from build123d import *

# Parameters (mm, degrees)
CROQUIS1_W                   = 15
CROQUIS1_H                   = 9
CROQUIS1_W_2                 = 13
CROQUIS1_H_2                 = 7
SALIENTE_EXTRUIR1_DEPTH      = 9
CROQUIS2_W                   = 15
CROQUIS2_H                   = 9
SALIENTE_EXTRUIR2_DEPTH      = 0.1
CROQUIS3_W                   = 3
CROQUIS3_H                   = 3.407555274
CORTAR_EXTRUIR1_DEPTH        = 7
CROQUIS4_W                   = 0.7
CROQUIS4_H                   = 0.7
SALIENTE_EXTRUIR3_DEPTH      = 3.5
SALIENTE_EXTRUIR3_DEPTH_BACK = 6


with BuildPart() as part:
    # Croquis1 → Saliente-Extruir1 (new body)
    with BuildSketch(Plane.XY):
        Rectangle(CROQUIS1_W, CROQUIS1_H)
        Rectangle(CROQUIS1_W_2, CROQUIS1_H_2, mode=Mode.SUBTRACT)
    extrude(amount=SALIENTE_EXTRUIR1_DEPTH)

    # Croquis2 → Saliente-Extruir2 (add)
    with BuildSketch(Plane(origin=(0, 0, 0), x_dir=(-1, 0, 0), z_dir=(0, 0, -1))):
        Rectangle(CROQUIS2_W, CROQUIS2_H)
    extrude(amount=SALIENTE_EXTRUIR2_DEPTH)

    # Croquis3 → Cortar-Extruir1 (cut)
    with BuildSketch(Plane.XY.offset(9)):
        with Locations((0, 3.5)):
            Rectangle(CROQUIS3_W, CROQUIS3_H)
    extrude(amount=-CORTAR_EXTRUIR1_DEPTH, mode=Mode.SUBTRACT)

    # Croquis4 → Saliente-Extruir3 (add, two sides)
    with BuildSketch(Plane(origin=(0, 0, -0.1), x_dir=(-1, 0, 0), z_dir=(0, 0, -1))) as saliente_extruir3_sk:
        with Locations((-2.15, 1.15)):
            Rectangle(CROQUIS4_W, CROQUIS4_H)
        with Locations((0.39, 1.15)):
            Rectangle(CROQUIS4_W, CROQUIS4_H)
        with Locations((2.93, 1.15)):
            Rectangle(CROQUIS4_W, CROQUIS4_H)
        with Locations((0.39, -1.39)):
            Rectangle(CROQUIS4_W, CROQUIS4_H)
        with Locations((2.93, -1.39)):
            Rectangle(CROQUIS4_W, CROQUIS4_H)
        with Locations((-2.15, -1.39)):
            Rectangle(CROQUIS4_W, CROQUIS4_H)
    extrude(amount=SALIENTE_EXTRUIR3_DEPTH)
    extrude(saliente_extruir3_sk.sketch, amount=-SALIENTE_EXTRUIR3_DEPTH_BACK)


solid = part.part
Here's how the part is built. I have some questions about the finished solid (model axes, mm). A direction names the side the tool comes from. Coordinates: 2 decimals unless noted, no trailing zeros. Loops run counter-clockwise (first coordinate to the right, second up) from the corner with the lowest first, then second, coordinate; pieces in that order, holes last.
1. For P1, Ø1, axis at x = 5, y = 2.5, coming from the -Z side; P2, Ø0.8, axis at y = 1, z = -2.5, coming from the -X side; P3, Ø0.8, axis at x = -0.5, z = 2.5, coming from the +Y side, each with a flat end and sliding along its axis, tell me the tip position at first contact or that it passes through.
2. For faces 1 (the flat face through (0, -4, 9)), 2 (the flat face through (0, 4, 2)), 3 (the flat face through (0, -3.5, 4)), which set-ups out of +Z, -Z, +X, -X, +Y, -Y let a thin tool reach every point of the face, with its end or its side?
3. Imagine slicing it at D-D, the plane z = -1.25. Please give me the cut outline in (x, y).
4. Imagine slicing it at B-B, the plane x = 6. Please give me the cut outline in (y, z), and give its area (3 significant figures).
5. If we mould it in two halves opening along Y, with no side actions, what happens to faces 4 (the flat face through (-6.5, 0, 4)), 5 (the flat face through (1.5, 4, 6)), 6 (the flat face through (0, -4.5, 5))? For each: pulls with the +Y half, pulls with the -Y half, needs draft (parallel to the pull), parting line crosses it, or undercut.
6. Imagine slicing it at A-A, the plane z = 0.75. Count the separate pieces of the cut face and the enclosed holes in it, and give its area (3 significant figures).
7. I need wall thicknesses on L1, parallel to X at y = 0, z = 4; L2, parallel to Y at x = -1, z = 1.25; L3, parallel to Y at x = 0.5, z = 3. Which ranges of each line are inside material? Lowest first, please.
Taken from the geometry:
1. P1: stops at z = -0.1
1. P2: stops at x = -3.28
1. P3: stops at y = 1.5
2. face 1: +Z, +X, -X, +Y, -Y
2. face 2: +Z, +Y
2. face 3: +Z
3. outline: (-3.28, -1.74) - (-2.58, -1.74) - (-2.58, -1.04) - (-3.28, -1.04) - close; (-3.28, 0.8) - (-2.58, 0.8) - (-2.58, 1.5) - (-3.28, 1.5) - close; (-0.74, -1.74) - (-0.04, -1.74) - (-0.04, -1.04) - (-0.74, -1.04) - close; (-0.74, 0.8) - (-0.04, 0.8) - (-0.04, 1.5) - (-0.74, 1.5) - close; (1.8, -1.74) - (2.5, -1.74) - (2.5, -1.04) - (1.8, -1.04) - close; (1.8, 0.8) - (2.5, 0.8) - (2.5, 1.5) - (1.8, 1.5) - close
4. outline: (-4.5, -0.1) - (4.5, -0.1) - (4.5, 9) - (3.5, 9) - (3.5, 0) - (-3.5, 0) - (-3.5, 9) - (-4.5, 9) - close
4. area: 18.9 mm2
5. face 4: undercut
5. face 5: needs draft
5. face 6: pulls with the -Y half
6. separate pieces: 7
6. enclosed holes: 1
6. area: 46.9 mm2
7. L1: x = -7.5 to -6.5, 6.5 to 7.5
7. L2: y = -4.5 to -3.5, 3.5 to 4.5
7. L3: y = -4.5 to -3.5
